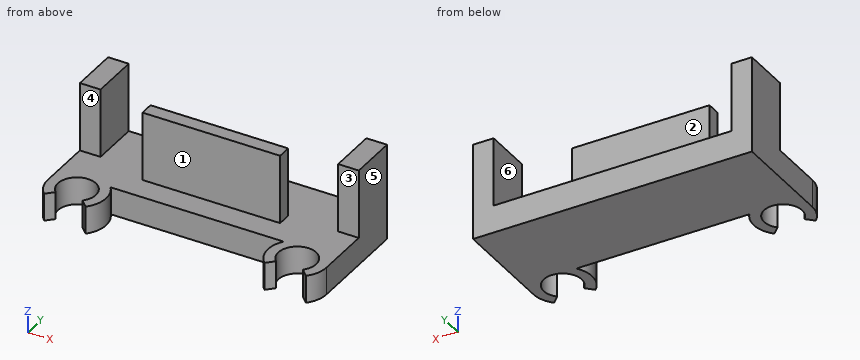
Autodesk Inventor part; units mm, degrees
ref_plane "YZ Plane" through (0, 0, 0) normal (1, 0, 0) x (0, 1, 0)
ref_plane "XZ Plane" through (0, 0, 0) normal (0, 1, 0) x (-1, 0, 0)
ref_plane "XY Plane" through (0, 0, 0) normal (0, 0, 1) x (1, 0, 0)
sketch "Sketch1" plane through (0, 0, 0) normal (0, 0, 1) x (1, 0, 0)
  line L0 (0, 0) -> (32, 0) construction
  line L1 (32, 0) -> (32, 15) construction
  line L2 (32, 15) -> (0, 15) construction
  line L3 (0, 15) -> (0, 0) construction
  circle A0 centre (0, 0) radius 2.75
  circle A1 centre (32, 0) radius 2.75
  line L4 (16, 15) -> (16, 0)
  line L5 (36.25, 0) -> (36.25, 15)
  line L6 (36.25, 15) -> (-4.25, 15)
  line L7 (-4.25, 15) -> (-4.25, 0)
  circle A2 centre (0, 0) radius 4.25
  circle A3 centre (32, 0) radius 4.25
  line L8 (3.4369, 2.5) -> (28.5631, 2.5)
  point P0 (0, 4.25)
  point P1 (32, 4.25)
  dimension "d0" = 32
  dimension "d2" = 15
  dimension "d4" = 5.5
  dimension "d6" = 1.5
  dimension "d7" = 1.5
  dimension "d10" = 5.5
  dimension "d11" = 2.5
extrude "Extrusion1" add sketch "Sketch1" along normal blind 4
sketch "Sketch2" plane through (0, 0, 4) normal (0, 0, 1) x (1, 0, 0)
  line L0 (-4.25, 15) -> (-4.25, 0)
  line L1 (3.4369, 2.5) -> (28.5631, 2.5)
  line L2 (36.25, 0) -> (36.25, 15)
  line L3 (0, 0) -> (-4.0526, -4.0526)
  line L4 (-4.0526, -4.0526) -> (0.938, -9.0431)
  line L5 (0.938, -9.0431) -> (4.9905, -4.9905)
  line L6 (4.9905, -4.9905) -> (0, 0)
  circle A0 centre (32, 0) radius 2.75 construction
  line L7 (32, 0) -> (27.2846, -4.7154)
  line L8 (27.2846, -4.7154) -> (32.2729, -9.7038)
  line L9 (32.2729, -9.7038) -> (36.9883, -4.9883)
  line L10 (36.9883, -4.9883) -> (32, 0)
  dimension "d24" = 45
extrude "Extrusion2" cut sketch "Sketch2" against normal through all
sketch "Sketch3" plane through (0, 0, 4) normal (0, 0, 1) x (1, 0, 0)
  line L0 (-4.25, 15) -> (-1.25, 15)
  line L1 (-1.25, 15) -> (-1.25, 8)
  line L2 (-1.25, 8) -> (-4.25, 8)
  line L3 (-4.25, 8) -> (-4.25, 15)
  line L4 (36.25, 15) -> (33.25, 15)
  line L5 (33.25, 15) -> (33.25, 8)
  line L6 (33.25, 8) -> (36.25, 8)
  line L7 (36.25, 8) -> (36.25, 15)
  line L8 (6, 6) -> (26, 6)
  line L9 (26, 6) -> (26, 8)
  line L10 (26, 8) -> (6, 8)
  line L11 (6, 8) -> (6, 6)
  line L12 (3.4369, 2.5) -> (28.5631, 2.5)
  point P0 (0, 0)
  point P1 (16, 6)
  point P2 (16, 2.5)
  dimension "d18" = 3
  dimension "d19" = 7
  dimension "d20" = 3
  dimension "d21" = 7
  dimension "d25" = 2
  dimension "d26" = 20
extrude "Extrusion3" add sketch "Sketch3" along normal blind 10
equation "\"d4\" = d10"
equation "\"d7\" = d6"
equation "\"d20\" = d18"
equation "\"d21\" = d19"
properties part number "switch lever"
Can you work these out from the model? Positions are in its coordinate system, mm. Face numbers are marked on the shaded views. A direction names the side the tool comes from. Coordinates: 2 decimals unless noted, no trailing zeros. Loops run counter-clockwise (first coordinate to the right, second up) from the corner with the lowest first, then second, coordinate; pieces in that order, holes last.
Item 1: Please list where these lines run through material, in increasing order: L1, parallel to X at y = 0, z = 2.25; L2, parallel to X at y = 1, z = 1.5; L3, parallel to X at y = 9.75, z = 6.
Answers below:
L1: x = -4.25 to -2.75, 2.75 to 4.25, 27.75 to 29.25, 34.75 to 36.25
L2: x = -4.25 to -2.56, 2.56 to 4.13, 27.87 to 29.44, 34.56 to 36.25
L3: x = -4.25 to -1.25, 33.25 to 36.25
Item 2: Which directions (+Z, -Z, +X, -X, +Y, -Y) give clear straight access to the entire face, cutting with the end or side of a thin tool? Please do the marked faces 1, 2 and 3.
Answers below:
face 1: +Z, +X, -X, -Y
face 2: +Z, +Y
face 3: +Z, +X, -Y
Item 3: Suppose I cut it at B-B (x = 16.5). Please give me the cut outline in (y, z), then the cut area to 3 significant figures.
Answers below:
outline: (2.5, 0) - (15, 0) - (15, 4) - (8, 4) - (8, 14) - (6, 14) - (6, 4) - (2.5, 4) - close
area: 70.0 mm2
Item 4: I'm going to push flat-ended pins straight in: pin 1 (2.5 mm diameter, centred on x = 35, z = 7.5, fed in from -Y); pin 2 (8 mm diameter, centred on x = 4.5, z = 11, fed in from -Y); pin 3 (5 mm diameter, centred on y = 4.5, z = 11, fed in from +X). Where does each tip first touch, or does it pass through?
Answers below:
pin 1: stops at y = 8
pin 2: stops at y = 6
pin 3: stops at x = 26
Item 5: Suppose I cut it at D-D (y = 10.25). Please give me the cut outline in (x, z), then the cut area to 3 significant figures.
Answers below:
outline: (-4.25, 0) - (36.25, 0) - (36.25, 14) - (33.25, 14) - (33.25, 4) - (-1.25, 4) - (-1.25, 14) - (-4.25, 14) - close
area: 222 mm2
Item 6: Suppose I cut it at A-A (z = 5.25). Please give me the cut outline in (x, y), then the cut area to 3 significant figures.
Answers below:
outline: (-4.25, 8) - (-1.25, 8) - (-1.25, 15) - (-4.25, 15) - close; (6, 6) - (26, 6) - (26, 8) - (6, 8) - close; (33.25, 8) - (36.25, 8) - (36.25, 15) - (33.25, 15) - close
area: 82.0 mm2
Item 7: If we mould it in two halves opening along X, with no side actions, what happens to the marked faces 4, 5 and 6? For each: released by +X, released by -X, zero draft, split by the parting line, or undercut.
Answers below:
face 4: zero draft
face 5: released by +X
face 6: undercut
Item 8: Suppose I cut it at C-C (y = -1.5). Please give me the cut outline in (x, z), then the cut area to 3 significant figures.
Answers below:
outline: (-3.98, 0) - (-2.3, 0) - (-2.3, 4) - (-3.98, 4) - close; (2.3, 0) - (3.98, 0) - (3.98, 4) - (2.3, 4) - close; (28.02, 0) - (29.7, 0) - (29.7, 4) - (28.02, 4) - close; (34.3, 0) - (35.98, 0) - (35.98, 4) - (34.3, 4) - close
area: 26.7 mm2
